```python
from build123d import *

# Parameters (mm, degrees)
BOSS_EXTRUDE1_DEPTH = 116
CUT_EXTRUDE1_DEPTH  = 120.398492453


with BuildPart() as part:
    # Sketch1 → Boss-Extrude1 (new body)
    with BuildSketch(Plane(origin=(0, 0, 0), x_dir=(0, 0, -1), z_dir=(1, 0, 0))):
        Polygon((0, 20), (0, 0), (20, 0), (20, 2), (2, 2), (2, 20), align=None)
    extrude(amount=BOSS_EXTRUDE1_DEPTH)

    # Sketch2 → Cut-Extrude1 (cut, through all)
    with BuildSketch(Plane.XZ):
        Polygon((0, 0), (4.251131233, -20), (0, -20), align=None)
    extrude(amount=-CUT_EXTRUDE1_DEPTH, mode=Mode.SUBTRACT)


solid = part.part
```
Verification items for the finished model (mm, model axes). A direction names the side the tool comes from. Coordinates: 2 decimals unless noted, no trailing zeros. Order: outer loops, then holes, each group sorted by start corner. A loop starts at its lowest first (then second) coordinate and runs counter-clockwise, first axis right, second up. Notation, with made-up numbers: (54, 8) -> (76, 8) arc R14 ccw to (76, 29) -> close; hole circle Ø8 at (46.5, 65). An arc over 180 degrees is marked (long way). Put each result on its own line as item: value. Start each with the question number.
1) Cross-section at A-A (x = 39). Enter the section's corners in (y, z), plus the area to 3 significant figures.
2) Material ranges on L1, parallel to Y at x = 82, z = -13.5; L2, parallel to Z at x = 82.5, y = 14.25; L3, parallel to X at y = 3.5, z = -1, recorded low to high.
3) Tool access check on faces 1 (the flat face through (59, 1, -20)), 2 (the flat face through (57, 2, -11)). Record the directions out of +Z, -Z, +X, -X, +Y, -Y that give a thin tool (end or side, any length) a straight path to the whole face; none if there is none.
4) Cross-section at C-C (z = -6.75). Enter the section's corners in (x, y).
5) Cross-section at B-B (y = 15). Enter the section's corners in (x, z), plus the area to 3 significant figures.
6) Go/stop test with flat-tipped pins: pin 1 (6 mm diameter, centred on x = 45.5, y = 11.5, fed in from -Z); pin 2 (4 mm diameter, centred on x = 62, z = -9, fed in from +Y). Record where each tip stops, or that it passes through.
Geometry check:
1. outline: (0, -20) -> (2, -20) -> (2, -2) -> (20, -2) -> (20, 0) -> (0, 0) -> close
1. area: 76.0 mm^2
2. L1: y = 0 to 2
2. L2: z = -2 to 0
2. L3: x = 0.21 to 116
3. face 1: -Z, +X, -X, +Y, -Y
3. face 2: -Z, +X, -X, +Y
4. outline: (1.43, 0) -> (116, 0) -> (116, 2) -> (1.43, 2) -> close
5. outline: (0, 0) -> (0.43, -2) -> (116, -2) -> (116, 0) -> close
5. area: 232 mm^2
6. pin 1: stops at z = -2
6. pin 2: stops at y = 2
